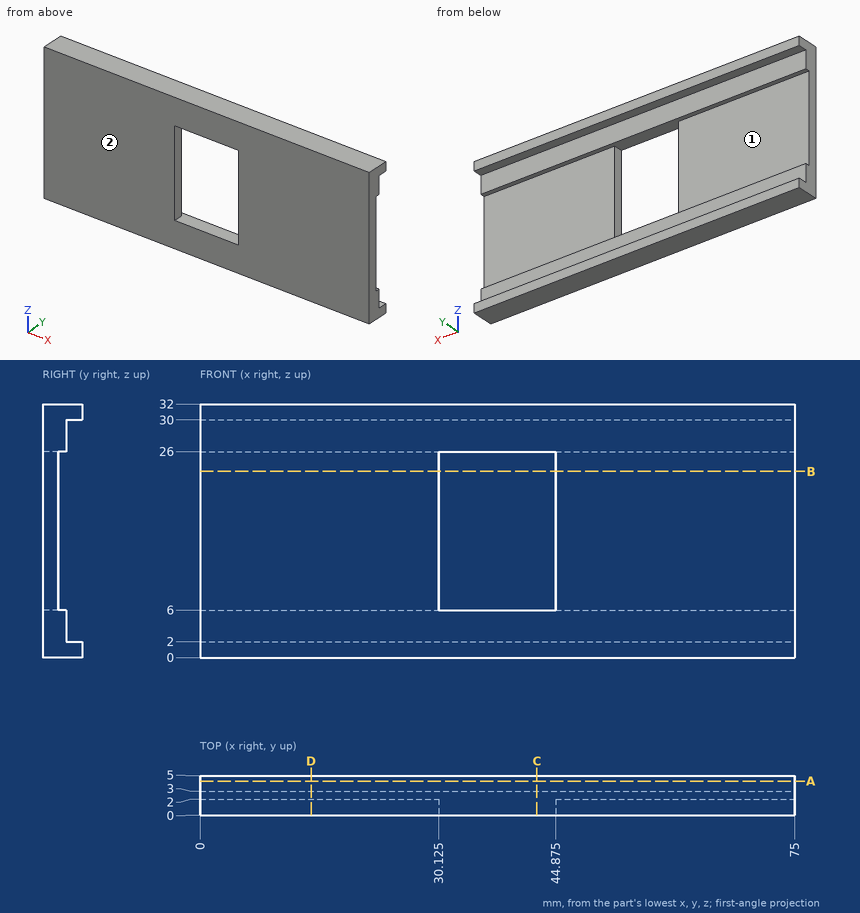
Verification items for this drawing (mm, ordinates from the low corner). Give positions to 0.01 mm unless a question says otherwise; leave off trailing zeros. Write each loop counter-clockwise with the first axis right and the second up, starting at its lowest first coordinate (ties: lowest second). Pieces come first, ordered by that corner, then holes. Notation, with made-up numbers: M 54.25,8 L 70.25,8 A21 cw 70.25,36 Z; hole C 18.5,44.5 d8. An arc over 180 degrees is marked long. Use one line per item in the form item = value.
(1) Draft check along Z on the marked faces 1 and 2. Enter one of: pulls with the +Z half, pulls with the -Z half, needs draft (parallel to the pull), parting line crosses it, or undercut.
Answer block:
face_1 = undercut
face_2 = needs draft
(2) Material ranges on line 1 along X through (y, z) = (1.8, 15.5) (3 decimals); line 2 along Z through (x, y) = (68.5, 4); line 3 along Z through (x, y) = (49, 2.1), recorded low to high.
Answer block:
line_1 = 0 to 30.125, 44.875 to 75
line_2 = 0 to 2, 30 to 32
line_3 = 0 to 6, 26 to 32
(3) Section check A-A on y = 4.3. Record the boundary of the cut face in (x, z), plus the area to 3 significant figures.
Answer block:
outline = M 0,0 L 75,0 L 75,2 L 0,2 Z; M 0,30 L 75,30 L 75,32 L 0,32 Z
area = 300 mm2
(4) Section check D-D on x = 14. Record the boundary of the cut face in (y, z).
Answer block:
outline = M 0,0 L 5,0 L 5,2 L 3,2 L 3,6 L 2,6 L 2,26 L 3,26 L 3,30 L 5,30 L 5,32 L 0,32 Z
(5) Section check C-C on x = 42.5. Record the boundary of the cut face in (y, z).
Answer block:
outline = M 0,0 L 5,0 L 5,2 L 3,2 L 3,6 L 0,6 Z; M 0,26 L 3,26 L 3,30 L 5,30 L 5,32 L 0,32 Z
(6) Depth check by flat-ended pin: P1, Ø1.2, axis at x = 25, z = 27.5, coming from the +Y side; P2, Ø10, axis at x = 35, z = 12, coming from the +Y side. Enter the tip coordinate at first touch or a pass-through.
Answer block:
P1 = 3
P2 = 2
(7) Section check B-B on z = 23.5. Record the boundary of the cut face in (x, y) (3 decimals), plus the area to 4 significant figures.
Answer block:
outline = M 0,0 L 30.125,0 L 30.125,2 L 0,2 Z; M 44.875,0 L 75,0 L 75,2 L 44.875,2 Z
area = 120.5 mm2
